Build history of the part. All positions in model axes, mm. Give positions to 0.01 mm unless a question says otherwise; leave off trailing zeros. Put each result on its own line as item: value. Start each with the question number.
Item 1: Flat gauge pins, fed straight in: pin 1 Ø1.5 at (x, z) = (9, 1.5) entering from -Y; pin 2 Ø4.5 at (x, y) = (-11, 0) entering from -Z; pin 3 Ø1 at (y, z) = (-16, 0.5) entering from +X. Where does each tip first touch, or does it go through?
Item 2: Drill centre lines: line 1 along Y through (x, z) = (0, 1.15); line 2 along X through (y, z) = (-2.5, 0.2); line 3 along Y through (x, z) = (0, 2.2). Where is each one in solid material? Low to high.
Item 3: Slice it at A-A, the plane x = 0. Give the number of separate pieces and of enclosed holes in the cut face, plus the area to 3 significant figures.
```python
from build123d import *

# Parameters (mm, degrees)
SKETCH_R             = 25
SKETCH_R_2           = 1.5
PAD_DEPTH            = 3
SKETCH002_R          = 2.25
POCKET_DEPTH         = 2
SKETCH001_R          = 5
POCKET001_DEPTH      = 1
SKETCH003_R          = 2.5
POCKET002_DEPTH      = 2
POCKET002_FACE17_R   = 5
POCKET002_FACE17_R_2 = 2.25
PAD001_DEPTH         = 1
CHAMFER_SIZE         = 0.4
CHAMFER001_SIZE      = 0.5
CHAMFER002_SIZE      = 0.4
CHAMFER003_SIZE      = 0.5
CHAMFER004_SIZE      = 0.5


with BuildPart() as part:
    # Sketch → Pad (new body)
    with BuildSketch(Plane.XY):
        Circle(SKETCH_R)
        with Locations((0, 11)):
            Circle(SKETCH_R_2, mode=Mode.SUBTRACT)
        with Locations((-11, 0)):
            Circle(SKETCH_R_2, mode=Mode.SUBTRACT)
        with Locations((0, -11)):
            Circle(SKETCH_R_2, mode=Mode.SUBTRACT)
        with Locations((11, 0)):
            Circle(SKETCH_R_2, mode=Mode.SUBTRACT)
    extrude(amount=PAD_DEPTH)

    # Sketch002 (on Face7 of Pad) → Pocket (cut)
    with BuildSketch(Plane.XY.offset(3)):
        Circle(SKETCH002_R)
    extrude(amount=-POCKET_DEPTH, mode=Mode.SUBTRACT)

    # Sketch001 (on Face7 of Pad) → Pocket001 (cut)
    with BuildSketch(Plane.XY.offset(3)):
        Circle(SKETCH001_R)
    extrude(amount=-POCKET001_DEPTH, mode=Mode.SUBTRACT)

    # Sketch003 (on Face2 of Pocket001) → Pocket002 (cut)
    with BuildSketch(Plane(origin=(0, 0, 0), x_dir=(1, 0, 0), z_dir=(0, 0, -1))):
        with Locations((0, 11)):
            Circle(SKETCH003_R)
        with Locations((11, 0)):
            Circle(SKETCH003_R)
        with Locations((0, -11)):
            Circle(SKETCH003_R)
        with Locations((-11, 0)):
            Circle(SKETCH003_R)
    extrude(amount=-POCKET002_DEPTH, mode=Mode.SUBTRACT)

    # Pocket002 Face17 → Pad001 (add)
    with BuildSketch(Plane(origin=(0, 0, 2), x_dir=(0, 1, 0), z_dir=(0, 0, 1))):
        Circle(POCKET002_FACE17_R)
        Circle(POCKET002_FACE17_R_2, mode=Mode.SUBTRACT)
    extrude(amount=PAD001_DEPTH)

    # Chamfer
    chamfer_edges = [part.edges().sort_by_distance(p)[0] for p in [
        (-1.5, -11, 3),
        (-12.5, 0, 3),
        (-1.5, 11, 3),
        (9.5, 0, 3),
    ]]
    chamfer(chamfer_edges, length=CHAMFER_SIZE)

    # Chamfer001
    chamfer001_edges = [part.edges().sort_by_distance(p)[0] for p in [
        (-2.25, 0, 3),
    ]]
    chamfer(chamfer001_edges, length=CHAMFER001_SIZE)

    # Chamfer002
    chamfer002_edges = [part.edges().sort_by_distance(p)[0] for p in [
        (9.5, 0, 2),
        (-1.5, -11, 2),
        (-12.5, 0, 2),
        (-1.5, 11, 2),
    ]]
    chamfer(chamfer002_edges, length=CHAMFER002_SIZE)

    # Chamfer003
    chamfer003_edges = [part.edges().sort_by_distance(p)[0] for p in [
        (-2.5, -11, 0),
        (8.5, 0, 0),
        (-13.5, 0, 0),
        (-2.5, 11, 0),
    ]]
    chamfer(chamfer003_edges, length=CHAMFER003_SIZE)

    # Chamfer004
    chamfer004_edges = [part.edges().sort_by_distance(p)[0] for p in [
        (-25, 0, 0),
        (-25, 0, 3),
    ]]
    chamfer(chamfer004_edges, length=CHAMFER004_SIZE)


solid = part.part
```
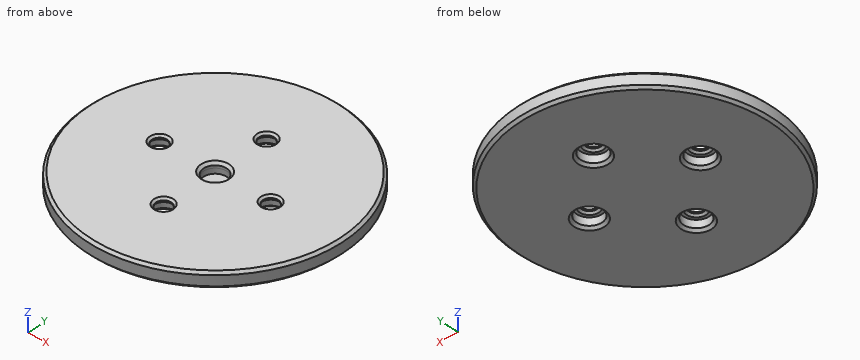
Values follow:
1. pin 1: y = -23.6
1. pin 2: z = 2
1. pin 3: x = 19.62
2. line 1: -25 to -13.5, -8.5 to -2.25, 2.25 to 8.5, 13.5 to 25
2. line 2: -24.57 to -12.26, -9.74 to 9.74, 12.26 to 24.57
2. line 3: -25 to -12.7, -9.3 to -2.25, 2.25 to 9.3, 12.7 to 25
3. separate pieces: 3
3. enclosed holes: 0
3. area: 113 mm2
